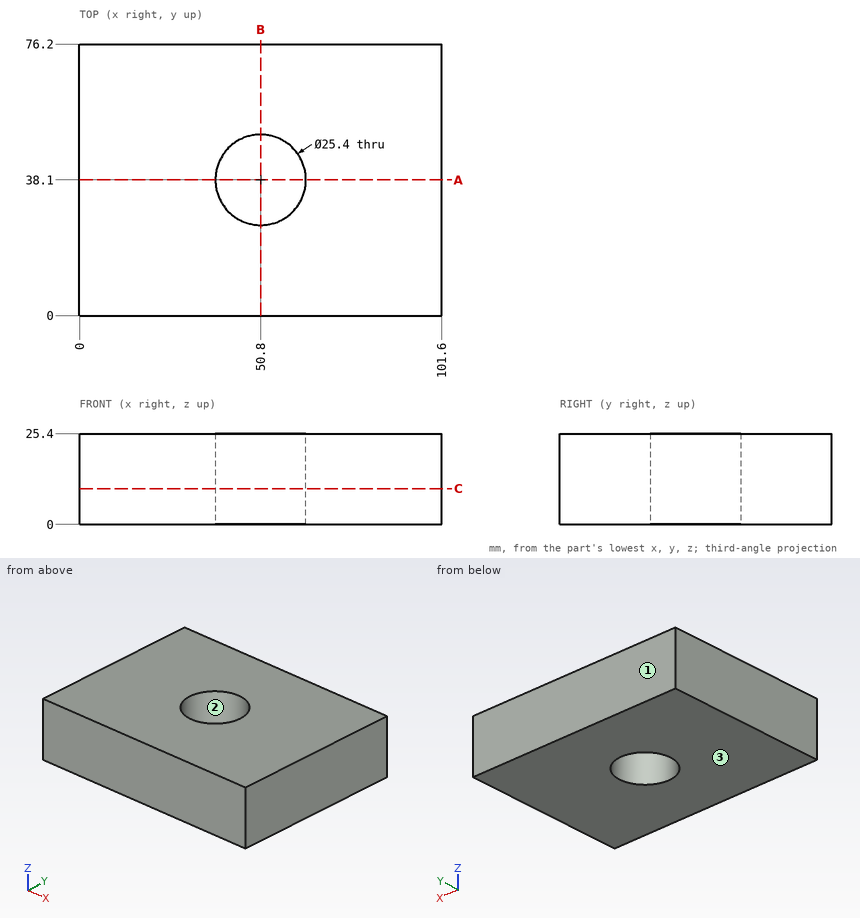
Source: three-view drawing plus pictorial views. Frame: mm from the lowest corner of the part. Coordinates: 2 decimals unless noted, no trailing zeros. Order: outer loops, then holes, each group sorted by start corner. A loop starts at its lowest first (then second) coordinate and runs counter-clockwise, first axis right, second up.
1) Section A-A (y = 38.1). Return loops of the section in (x, z), then the cut area to 3 significant figures.
Result sheet:
outline: (0, 0) - (38.1, 0) - (38.1, 25.4) - (0, 25.4) - close; (63.5, 0) - (101.6, 0) - (101.6, 25.4) - (63.5, 25.4) - close
area: 1,940 mm2
2) Draft query along Y for the marked faces 1, 2 and 3. Return one class per face: released by +Y, released by -Y, zero draft, split by the parting line, or undercut.
Result sheet:
face 1: released by +Y
face 2: undercut
face 3: zero draft
3) Section C-C (z = 10). Return loops of the section in (x, y), then the cut area to 3 significant figures.
Result sheet:
outline: (0, 0) - (101.6, 0) - (101.6, 76.2) - (0, 76.2) - close; hole circle Ø25.4 at (50.8, 38.1)
area: 7,240 mm2
4) Section B-B (x = 50.8). Return loops of the section in (y, z).
Result sheet:
outline: (0, 0) - (25.4, 0) - (25.4, 25.4) - (0, 25.4) - close; (50.8, 0) - (76.2, 0) - (76.2, 25.4) - (50.8, 25.4) - close
5) Ray query, probe 1 along Y at (x, z) = (50.8, 7.5); probe 2 along Y at (x, z) = (49.5, 10.75); probe 3 along X at (y, z) = (36, 2.5). Return the intervals inside material, ascending.
Result sheet:
probe 1: y = 0 to 25.4, 50.8 to 76.2
probe 2: y = 0 to 25.47, 50.73 to 76.2
probe 3: x = 0 to 38.27, 63.33 to 101.6
6) First-contact query: P1, Ø4, axis at y = 13.5, z = 21.5, coming from the -X side. Flat tip, straight axial feed; report the tip coordinate or a pass-through.
Result sheet:
P1: stops at x = 0
